Here's how the part is built. I have some questions about the finished solid (model axes, mm). A direction names the side the tool comes from. Give positions to 0.01 mm unless a question says otherwise; leave off trailing zeros. Loops run counter-clockwise (first coordinate to the right, second up) from the corner with the lowest first, then second, coordinate; pieces in that order, holes last. Notation, with made-up numbers: (42.25, 7) - (90.25, 7) arc R14 ccw to (90.25, 15) - close; hole circle Ø2 at (47.5, 81.5). An arc over 180 degrees is marked (long way). Put each result on its own line as item: value. Start each with the question number.
from build123d import *

# Parameters (mm, degrees)
CROQUIS1_W              = 31
CROQUIS1_H              = 47.5
CROQUIS1_R              = 1.5
SALIENTE_EXTRUIR1_DEPTH = 5
CORTAR_EXTRUIR1_DEPTH   = 10
CORTAR_EXTRUIR2_START   = -4
CROQUIS4_R              = 1.5
CORTAR_EXTRUIR2_DEPTH   = 4
SALIENTE_EXTRUIR2_START = -6
CROQUIS5_R              = 2.355
SALIENTE_EXTRUIR2_DEPTH = 10


with BuildPart() as part:
    # Croquis1 → Saliente-Extruir1 (new, symmetric)
    with BuildSketch(Plane.XY):
        Rectangle(CROQUIS1_W, CROQUIS1_H)
        Circle(CROQUIS1_R, mode=Mode.SUBTRACT)
    extrude(amount=SALIENTE_EXTRUIR1_DEPTH, both=True)

    # Croquis2 → Cortar-Extruir1 (cut)
    with BuildSketch(Plane.XY.offset(5)):
        with BuildLine():
            ThreePointArc((-15.5, -8.75), (-26.106601718, -34.356601718), (-0.5, -23.75))
            Line((-0.5, -23.75), (-15.5, -23.75))
            Line((-15.5, -23.75), (-15.5, -8.75))
        make_face()
        with BuildLine():
            Line((-15.5, -23.75), (-0.5, -23.75))
            ThreePointArc((-0.5, -23.75), (-0.864332185, -20.464086488), (-1.939630348, -17.337794848))
            ThreePointArc((-1.939630348, -17.337794848), (-7.474511768, -11.077528314), (-15.5, -8.75))
            Line((-15.5, -8.75), (-15.5, -23.75))
        make_face()
        with BuildLine():
            Line((-0.5, -23.75), (8.68, -23.75))
            ThreePointArc((8.68, -23.75), (2.477320667, -22.022622308), (-1.939630348, -17.337794848))
            ThreePointArc((-1.939630348, -17.337794848), (-0.864332185, -20.464086488), (-0.5, -23.75))
        make_face()
        with BuildLine():
            Line((8.68, -23.75), (15.5, -23.75))
            Line((15.5, -23.75), (15.5, -21.623580911))
            ThreePointArc((15.5, -21.623580911), (12.251906289, -23.206067627), (8.68, -23.75))
        make_face()
        with BuildLine():
            ThreePointArc((-1.706345602, 17.75), (6.388766151, 22.206978995), (15.5, 23.75))
            Line((15.5, 23.75), (-15.5, 23.75))
            Line((-15.5, 23.75), (-15.5, -5.75))
            ThreePointArc((-15.5, -5.75), (-4.526914837, 3.607383252), (-1.706345602, 17.75))
        make_face()
        with BuildLine():
            ThreePointArc((15.5, 23.75), (8.791561976, 11.25), (15.5, -1.25))
            Line((15.5, -1.25), (15.5, 23.75))
        make_face()
    extrude(amount=-CORTAR_EXTRUIR1_DEPTH, mode=Mode.SUBTRACT)

    # Croquis4 → Cortar-Extruir2 (cut)
    with BuildSketch(Plane.XY.offset(5).offset(CORTAR_EXTRUIR2_START)):
        with BuildLine():
            ThreePointArc((0.741753077, -15.99078245), (-3.792394766, -10.077692964), (-10.332847598, -6.50759483))
            ThreePointArc((-10.332847598, -6.50759483), (-1.276413132, 3.29347854), (1.447897595, 16.357098845))
            ThreePointArc((1.447897595, 16.357098845), (4.511231243, 18.167637942), (7.803157135, 19.518670428))
            ThreePointArc((7.803157135, 19.518670428), (6.178453275, 7.53807302), (12.5, -2.767868174))
            Line((12.5, -2.767868174), (12.5, -19.899085838))
            ThreePointArc((12.5, -19.899085838), (5.841215353, -20.290567998), (0.741753077, -15.99078245))
        make_face()
        Circle(CROQUIS4_R, mode=Mode.SUBTRACT)
    cortar_extruir2 = extrude(amount=CORTAR_EXTRUIR2_DEPTH, mode=Mode.SUBTRACT)

    # Simetría1: Cortar-Extruir2 across plane
    add(cortar_extruir2.mirror(Plane.XY), mode=Mode.SUBTRACT)

    # Croquis5 → Saliente-Extruir2 (add)
    with BuildSketch(Plane.XY.offset(1).offset(SALIENTE_EXTRUIR2_START)):
        with BuildLine():
            ThreePointArc((-4.313183402, -1.283140267), (0.648334286, -4.453050938), (4.5, 0))
            ThreePointArc((4.5, 0), (2.91581216, 3.427541312), (-0.721350866, 4.441807394))
            ThreePointArc((-0.721350866, 4.441807394), (-2.322917222, 1.457398417), (-4.313183402, -1.283140267))
        make_face()
        with Locations(Location((0, 0, 0), (0, 0, 180))):
            Circle(CROQUIS5_R, mode=Mode.SUBTRACT)
    extrude(amount=SALIENTE_EXTRUIR2_DEPTH)


solid = part.part
1) Suppose I cut it at D-D on x = 6.5. Please give me the cut outline in (y, z), plus the area to 3 significant figures.
2) Which directions (+Z, -Z, +X, -X, +Y, -Y) give clear straight access to the entire face, cutting with the end or side of a thin tool? Please do faces 5 (the cylindrical face through (1.87, 1.43, 2.97)), 6 (the flat face through (-2, 0, -1)), 7 (the cylindrical face through (6.266, 22.164, 0.07)).
3) I'm going to push flat-ended pins straight in: P1, Ø1.5, axis at x = 0, z = -3.5, coming from the -Y side; P2, Ø5, axis at x = 2.5, z = 0, coming from the -Y side; P3, Ø1.5, axis at x = 7.5, z = 3, coming from the +Y side. Where does each tip first touch, or does it pass through?
4) I need wall thicknesses on line 1 (X direction, y = 2, z = -2.5); line 2 (Y direction, x = 10.5, z = 3.5); line 3 (Y direction, x = 4, z = 3). Which ranges of each line are inside material? Lowest first, please.
5) Thinking about a two-plate mould opening in X: for faces 1 (the cylindrical face through (8.793, 11.457, 0.07)), 2 (the flat face through (2, -3, 5)), 3 (the flat face through (12.5, -11, 3)), 4 (the cylindrical face through (-7.375, -11.141, 0.07)), which applies, pulls with the +X half, pulls with the -X half, needs draft (parallel to the pull), parting line crosses it, or undercut?
6) Suppose I cut it at A-A on z = -4. Please give me the cut outline in (x, y) (3 decimals).
7) Suppose I cut it at C-C on y = 9. Please give me the cut outline in (x, z).
Ans:
1. outline: (-23.55, -5) - (-20.48, -5) - (-20.48, -1) - (6.25, -1) - (6.25, -5) - (16.25, -5) - (16.25, -1) - (19.05, -1) - (19.05, -5) - (22.25, -5) - (22.25, 5) - (19.05, 5) - (19.05, 1) - (16.25, 1) - (16.25, 5) - (6.25, 5) - (6.25, 1) - (-20.48, 1) - (-20.48, 5) - (-23.55, 5) - close
1. area: 222 mm²
2. face 5: +Z
2. face 6: -Z
2. face 7: +Z, -Z, -X, +Y
3. P1: stops at y = -20.76
3. P2: stops at y = -23.17
3. P3: stops at y = 22.78
4. line 1: x = -5.57 to -1.24, 1.24 to 4.03, 8.35 to 11.98
4. line 2: y = -23.61 to -20.56, -0.89 to 4.3, 18.2 to 23.29
4. line 3: y = -22.8 to -19.44, -2.06 to 2.06, 17.91 to 21.25
5. face 1: pulls with the +X half
5. face 2: needs draft
5. face 3: undercut
5. face 4: pulls with the -X half
6. outline: (-15.5, -8.75) arc R15 cw to (-1.94, -17.338) arc R12 ccw to (15.5, -21.624) - (15.5, -1.25) arc R15 cw to (15.5, 23.75) arc R27.672 ccw to (-1.706, 17.75) arc R22 cw to (-15.5, -5.75) - close; hole (-10.333, -6.508) arc R18 cw to (0.742, -15.991) arc R9 ccw to (12.5, -19.899) - (12.5, -2.768) arc R18 cw to (7.803, 19.519) arc R24.672 ccw to (1.448, 16.357) arc R25 cw to (-0.721, 4.442) arc R4.5 cw (long way) to (-4.313, -1.283) arc R25 cw to start; hole circle Ø4.71 at (0, 0)
7. outline: (-2.26, -5) - (0.83, -5) - (0.83, -1) - (5.93, -1) - (5.93, -5) - (8.96, -5) - (8.96, 5) - (5.93, 5) - (5.93, 1) - (0.83, 1) - (0.83, 5) - (-2.26, 5) - close
